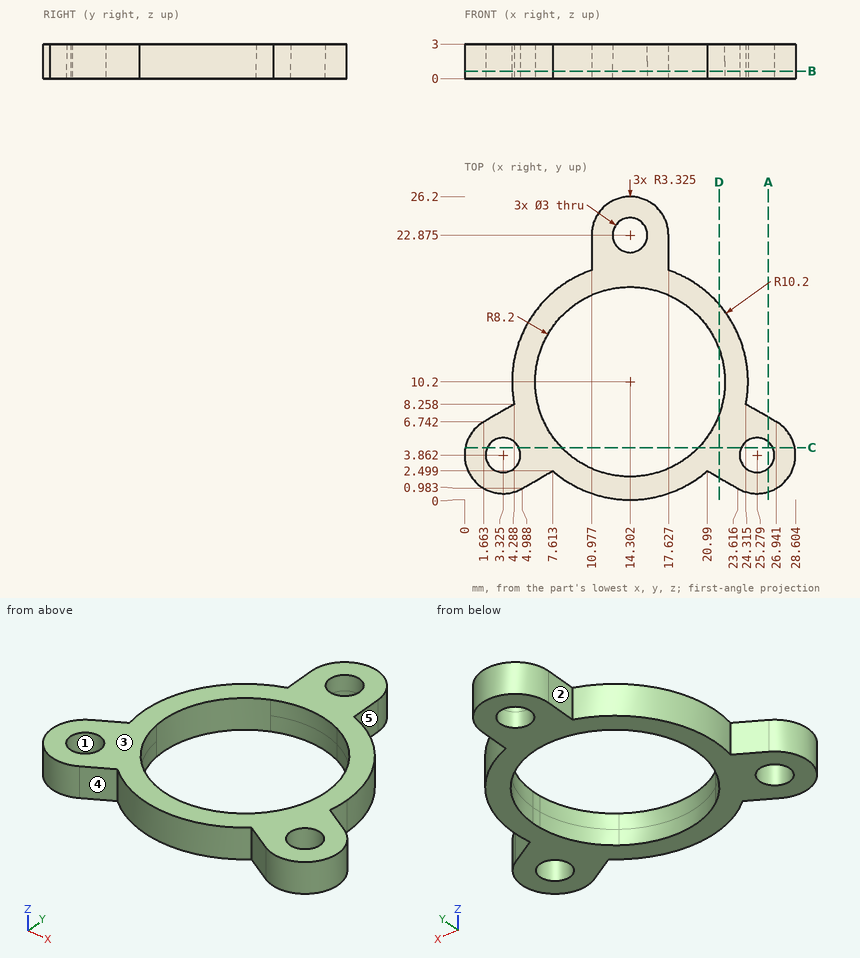
Geometry: see drawing. Coordinates: mm, zero at the bounding-box minimum. A direction names the side the tool comes from. Round coordinates to 2 decimals unless told otherwise and drop trailing zeros. Write each loop counter-clockwise with the first axis right and the second up, starting at its lowest first coordinate (ties: lowest second). Pieces come first, ordered by that corner, then holes.
Item 1: Material intervals for L1, parallel to X at y = 4.75, z = 2.8 (1 decimal); L2, parallel to Y at x = 14, z = 2.5 (1 decimal); L3, parallel to X at y = 13, z = 2.2 (1 decimal), sorted ascending.
Item 2: Section query A-A (x = 26.25). Return loops of the section in (y, z) (1 decimal).
Item 3: Section query B-B (z = 0.65). Give the number of separate pieces and of enclosed holes in the cut face.
Item 4: Section query C-C (y = 4.5). Return loops of the section in (x, z).
Item 5: Set-up query: the marked faces 1, 2, 3, 4 and 5. Return all of +Z, -Z, +X, -X, +Y, -Y with unobstructed straight access to the full face (end or side cutting, diameter ignored); none if empty.
Item 6: Section query D-D (x = 22). Return loops of the section in (y, z) (1 decimal).
Item 7: Pin query (flat end, axial travel): P1, Ø1.8, axis at x = 3.33, y = 3.86, coming from the +Z side; P2, Ø0.9, axis at y = 21.5, z = 1.5, coming from the +X side. Return the tip coordinate at first contact, or that it passes through.
Completed:
1. L1: x = 0.1 to 2.1, 4.5 to 8.2, 20.4 to 24.1, 26.5 to 28.5
1. L2: y = 0 to 2, 18.4 to 21.4, 24.3 to 26.2
1. L3: x = 4.5 to 6.6, 22 to 24.1
2. outline: (0.7, 0) - (2.7, 0) - (2.7, 3) - (0.7, 3) - close; (5, 0) - (7.1, 0) - (7.1, 3) - (5, 3) - close
3. separate pieces: 1
3. enclosed holes: 4
4. outline: (0.06, 0) - (1.97, 0) - (1.97, 3) - (0.06, 3) - close; (4.68, 0) - (8.41, 0) - (8.41, 3) - (4.68, 3) - close; (20.2, 0) - (23.92, 0) - (23.92, 3) - (20.2, 3) - close; (26.64, 0) - (28.54, 0) - (28.54, 3) - (26.64, 3) - close
5. face 1: +Z, -Z
5. face 2: +Z, -Z, -X, +Y
5. face 3: +Z, +X, -X, +Y, -Y
5. face 4: +Z, -Z, -Y
5. face 5: +Z, -Z, +X, +Y
6. outline: (1.9, 0) - (7.4, 0) - (7.4, 3) - (1.9, 3) - close; (13, 0) - (16.9, 0) - (16.9, 3) - (13, 3) - close
7. P1: passes through
7. P2: stops at x = 17.63
